Work out the finished part from the listing and answer in its coordinate system (mm). Face numbers are marked on the shaded views. A direction names the side the tool comes from. Give positions to 0.01 mm unless a question says otherwise; leave off trailing zeros. Order: outer loops, then holes, each group sorted by start corner. A loop starts at its lowest first (then second) coordinate and runs counter-clockwise, first axis right, second up. Notation, with made-up numbers: (25.5, 46.5) -> (42.5, 46.5) arc R17 ccw to (42.5, 53.5) -> close; hole circle Ø5 at (4, 39.5). An arc over 180 degrees is marked (long way). Use a Markdown table: item, result. Add a question column.
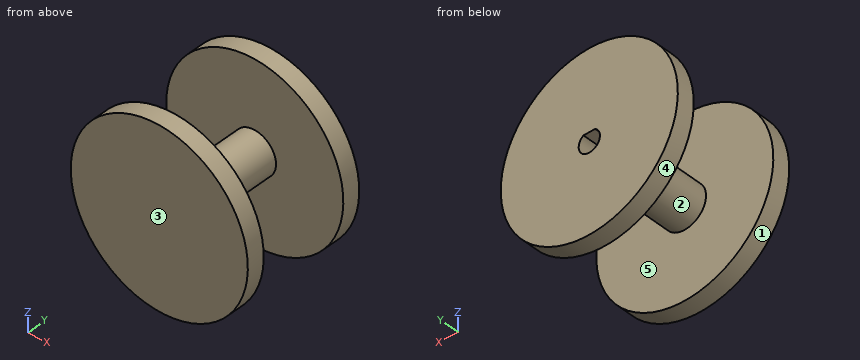
```python
from build123d import *

# Parameters (mm, degrees)
SKETCH1_R           = 25
BOSS_EXTRUDE1_DEPTH = 5
SKETCH2_R           = 6
BOSS_EXTRUDE2_DEPTH = 25
SKETCH3_R           = 25
BOSS_EXTRUDE3_DEPTH = 5
CUT_EXTRUDE1_DEPTH  = 10


with BuildPart() as part:
    # Sketch1 → Boss-Extrude1 (new body)
    with BuildSketch(Plane(origin=(0, 0, 0), x_dir=(1, 0, 0), z_dir=(0, 1, 0))):
        with Locations(Location((0, 0, 0), (0, 0, 270))):
            Circle(SKETCH1_R)
    extrude(amount=BOSS_EXTRUDE1_DEPTH)

    # Sketch2 → Boss-Extrude2 (add)
    with BuildSketch(Plane(origin=(0, 5, 0), x_dir=(1, 0, 0), z_dir=(0, 1, 0))):
        with Locations(Location((0, 0, 0), (0, 0, 270))):
            Circle(SKETCH2_R)
    extrude(amount=BOSS_EXTRUDE2_DEPTH)

    # Sketch3 → Boss-Extrude3 (add)
    with BuildSketch(Plane(origin=(0, 30, 0), x_dir=(1, 0, 0), z_dir=(0, 1, 0))):
        with Locations(Location((0, 0, 0), (0, 0, 270))):
            Circle(SKETCH3_R)
    extrude(amount=BOSS_EXTRUDE3_DEPTH)

    # Sketch4 → Cut-Extrude1 (cut)
    with BuildSketch(Plane(origin=(0, 35, 0), x_dir=(1, 0, 0), z_dir=(0, 1, 0))):
        with BuildLine():
            Line((0, -2.5), (-1.658312395, -2.5))
            ThreePointArc((-1.658312395, -2.5), (0, 3), (1.658312395, -2.5))
            Line((1.658312395, -2.5), (0, -2.5))
        make_face()
    extrude(amount=-CUT_EXTRUDE1_DEPTH, mode=Mode.SUBTRACT)


solid = part.part
```
1) Which of the six approach directions +Z, -Z, +X, -X, +Y, -Y give full straight-line access (tool end or side, diameter ignored) to the marked faces 4 and 5?
2) The part is cut by section B-B, the plane z = 0. Determine the outline of the cut face in (x, y).
3) Determine the mould class of the marked faces 1, 2 and 3 for opening direction Y: released by +Y, released by -Y, zero draft, split by the parting line, or undercut.
4) The part is cut by section C-C, the plane x = 0. Determine the outline of the cut face in (y, z), then the cut area to 3 significant figures.
5) Straight lines are drawn through the part: line 1 (Y direction, x = -9, z = 17.5); line 2 (X direction, y = 31, z = 0); line 3 (X direction, y = 29.75, z = 0). For each, find the intervals that lie inside material, in ascending order.
6) The part is cut by section D-D, the plane y = 11.5. Determine the outline of the cut face in (x, z).
7) Flat-ended cylindrical pins translate along their axes: pin 1 (6 mm diameter, centred on x = 1, z = 1, fed in from +Y); pin 2 (5 mm diameter, centred on x = -1, y = 13.5, fed in from -Z); pin 3 (10 mm diameter, centred on y = 26.5, z = 2.5, fed in from -X); pin 4 (1 mm diameter, centred on y = 31, z = -4.5, fed in from -X). Find the tip coordinate at first contact, or state that the pin passes through.
8) The part is cut by section A-A, the plane x = 8.5. Determine the outline of the cut face in (y, z), then the cut area to 3 significant figures.
A:
| question | item | result |
|---|---|---|
| 1 | face 4 | +Y, -Y |
| 1 | face 5 | none |
| 2 | outline | (-25, 0) -> (25, 0) -> (25, 5) -> (6, 5) -> (6, 30) -> (25, 30) -> (25, 35) -> (3, 35) -> (3, 25) -> (-3, 25) -> (-3, 35) -> (-25, 35) -> (-25, 30) -> (-6, 30) -> (-6, 5) -> (-25, 5) -> close |
| 3 | face 1 | zero draft |
| 3 | face 2 | undercut |
| 3 | face 3 | released by -Y |
| 4 | outline | (0, -25) -> (5, -25) -> (5, -6) -> (30, -6) -> (30, -25) -> (35, -25) -> (35, -3) -> (25, -3) -> (25, 2.5) -> (35, 2.5) -> (35, 25) -> (30, 25) -> (30, 6) -> (5, 6) -> (5, 25) -> (0, 25) -> close |
| 4 | area | 745 mm^2 |
| 5 | line 1 | 0 to 5, 30 to 35 |
| 5 | line 2 | -25 to -3, 3 to 25 |
| 5 | line 3 | -6 to -3, 3 to 6 |
| 6 | outline | circle Ø12 at (0, 0) |
| 7 | pin 1 | y = 35 |
| 7 | pin 2 | z = -6 |
| 7 | pin 3 | x = -25 |
| 7 | pin 4 | x = -24.68 |
| 8 | outline | (0, -23.51) -> (5, -23.51) -> (5, 23.51) -> (0, 23.51) -> close; (30, -23.51) -> (35, -23.51) -> (35, 23.51) -> (30, 23.51) -> close |
| 8 | area | 470 mm^2 |
